from build123d import *

# Parameters (mm, degrees)
SKETCH2_R           = 6.57086473
CUT_EXTRUDE3_DEPTH  = 5
SKETCH3_W           = 0.4
SKETCH3_H           = 2
BOSS_EXTRUDE2_DEPTH = 5.8


with BuildPart() as part:
    # Sketch1 → Revolve2 (revolve)
    with BuildSketch(Plane.XY, mode=Mode.PRIVATE) as revolve2_sk:
        Polygon((0, 20.6), (3, 20.6), (3, 15), (2.446439684, 15), (2.446439684, 11.9), (3.5, 11.9), (3.5, 11), (5.715, 11), (5.715, 9), (4, 9), (4, 6), (3.444705053, 6), (3.444705053, 0), (0, 0), align=None)
    revolve(revolve2_sk.sketch.rotate(Axis((0, 22.726966954, 0), (0, -1, 0)), 90), axis=Axis((0, 22.726966954, 0), (0, -1, 0)))

    # Sketch2 → Cut-Extrude3 (cut)
    with BuildSketch(Plane(origin=(0, 11, 0), x_dir=(1, 0, 0), z_dir=(0, 1, 0))):
        Circle(SKETCH2_R)
        Polygon((5.715, 0), (2.8575, 4.949335183), (-2.8575, 4.949335183), (-5.715, 0), (-2.8575, -4.949335183), (2.8575, -4.949335183), align=None, mode=Mode.SUBTRACT)
    extrude(amount=-CUT_EXTRUDE3_DEPTH, mode=Mode.SUBTRACT)

    # Sketch3 → Boss-Extrude2 (add)
    with BuildSketch(Plane.XZ):
        with Locations((-2.05, 0)):
            Rectangle(SKETCH3_W, SKETCH3_H)
        with Locations((2.05, 0)):
            Rectangle(SKETCH3_W, SKETCH3_H)
    extrude(amount=BOSS_EXTRUDE2_DEPTH)


solid = part.part
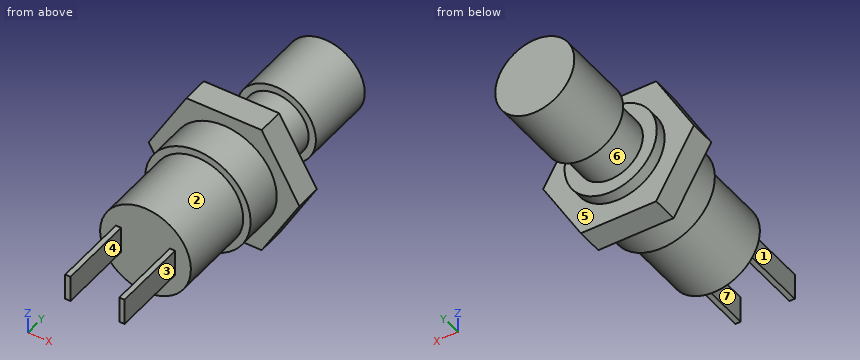
Read the model definition and answer for the solid it produces. Units are mm, in the model's axes. Face numbers are marked on the shaded views. A direction names the side the tool comes from. Round coordinates to 2 decimals unless told otherwise and drop trailing zeros. Loops run counter-clockwise (first coordinate to the right, second up) from the corner with the lowest first, then second, coordinate; pieces in that order, holes last.
Q1. Each of these flat-tipped pins is pushed along its axis until it touches: pin 1 (1 mm diameter, centred on y = -4, z = 0.5, fed in from +X); pin 2 (4 mm diameter, centred on y = -1, z = 0.5, fed in from +X); pin 3 (2 mm diameter, centred on x = -2.5, z = 4, fed in from +Y). Where does it stop, or does it pass through?
Q2. Section D-D on y = 18.75 is taken. Write down the section's boundary in (x, z).
Q3. Determine the mould class of the marked faces 5, 6 and 7 for opening direction Y: released by +Y, released by -Y, zero draft, split by the parting line, or undercut.
Q4. Which of the six approach directions +Z, -Z, +X, -X, +Y, -Y give full straight-line access (tool end or side, diameter ignored) to the marked faces 1, 2, 3 and 4?
Q5. Section B-B on y = 10.5 is taken. Write down the section's boundary in (x, z) (1 decimal).
Q6. Section A-A on x = 0 is taken. Write down the section's boundary in (y, z).
Q7. Consider probe 1 along Y at (x, z) = (-2, 3); probe 2 along Y at (x, z) = (1, 4.5); probe 3 along Z at (x, y) = (-1, 0.75). Determine where each line is inside the solid, lowest interval first.
Output:
1. pin 1: stops at x = 2.25
1. pin 2: stops at x = 3.44
1. pin 3: stops at y = 11
2. outline: circle Ø6 at (0, 0)
3. face 5: released by +Y
3. face 6: undercut
3. face 7: zero draft
4. face 1: +Z, -Z, -X, -Y
4. face 2: -Y
4. face 3: +Z, -Z, +X, -Y
4. face 4: +Z, -Z, -Y
5. outline: (-5.7, 0) - (-2.9, -4.9) - (2.9, -4.9) - (5.7, 0) - (2.9, 4.9) - (-2.9, 4.9) - close
6. outline: (0, -3.44) - (6, -3.44) - (6, -4) - (9, -4) - (9, -4.95) - (11, -4.95) - (11, -3.5) - (11.9, -3.5) - (11.9, -2.45) - (15, -2.45) - (15, -3) - (20.6, -3) - (20.6, 3) - (15, 3) - (15, 2.45) - (11.9, 2.45) - (11.9, 3.5) - (11, 3.5) - (11, 4.95) - (9, 4.95) - (9, 4) - (6, 4) - (6, 3.44) - (0, 3.44) - close
7. probe 1: y = 6 to 11
7. probe 2: y = 9 to 11
7. probe 3: z = -3.3 to 3.3
